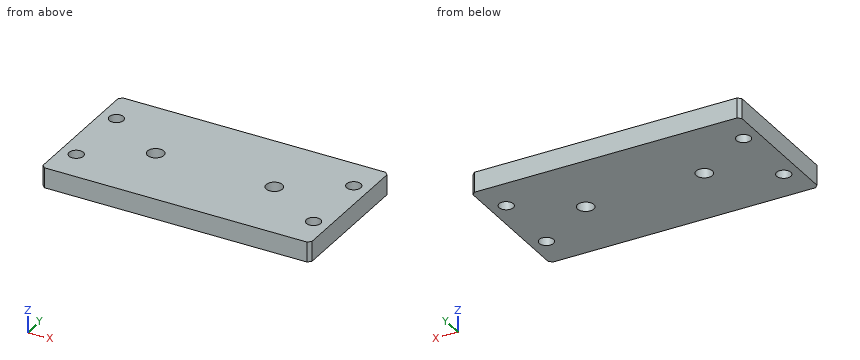
```python
from build123d import *

# Parameters (mm, degrees)
F0_W     = 170
F0_H     = 88
F0_R     = 4.5
F1_DEPTH = 6.35
F2_SIZE  = 2
F4_D     = 10.3


with BuildPart() as f1:
    # F0 (on Top) → F1 (new body, symmetric)
    with BuildSketch(Plane.XY):
        Rectangle(F0_W, F0_H)
        with Locations((-75, -22.5)):
            Circle(F0_R, mode=Mode.SUBTRACT)
        with Locations((75, -22.5)):
            Circle(F0_R, mode=Mode.SUBTRACT)
        with Locations((-75, 22.5)):
            Circle(F0_R, mode=Mode.SUBTRACT)
        with Locations((75, 22.5)):
            Circle(F0_R, mode=Mode.SUBTRACT)
    extrude(amount=F1_DEPTH, both=True)

    # F2
    f2_edges = [f1.edges().sort_by_distance(p)[0] for p in [
        (85, 44, 0),
        (85, -44, 0),
        (-85, 44, 0),
        (-85, -44, 0),
    ]]
    chamfer(f2_edges, length=F2_SIZE)

    # F4 (through all)
    with Locations(Plane.XY.offset(6.35)):
        with Locations((-37.5, 0), (37.5, 0)):
            Hole(F4_D / 2)


solid = f1.part
```
Source: CAD feature listing. Evaluate the final solid. Frame: model axes, mm. Give positions to 0.01 mm unless a question says otherwise; leave off trailing zeros. Order: outer loops, then holes, each group sorted by start corner. A loop starts at its lowest first (then second) coordinate and runs counter-clockwise, first axis right, second up.
(1) Section query A-A (x = 37.5). Return the cut outline in (y, z).
(2) Section query B-B (y = 0). Return the cut outline in (x, z).
(3) Contact query for flat-ended pins moving along their axis: P1, Ø8, axis at x = -75, y = 22.5, coming from the -Z side; P2, Ø10.5, axis at x = 75, y = -22.5, coming from the +Z side. Output: stop coordinate, or through.
(4) Section query C-C (z = -3.25). Return the cut outline in (x, y), plus the area to 3 significant figures.
(5) Material intervals for line 1 along Y through (x, z) = (-75, -1.25); line 2 along Y through (x, z) = (37.5, -1); line 3 along X through (y, z) = (18.5, -3), sorted ascending.
(6) Section query D-D (x = 75). Return the cut outline in (y, z).
Outcome:
1. outline: (-44, -6.35) - (-5.15, -6.35) - (-5.15, 6.35) - (-44, 6.35) - close; (5.15, -6.35) - (44, -6.35) - (44, 6.35) - (5.15, 6.35) - close
2. outline: (-85, -6.35) - (-42.65, -6.35) - (-42.65, 6.35) - (-85, 6.35) - close; (-32.35, -6.35) - (32.35, -6.35) - (32.35, 6.35) - (-32.35, 6.35) - close; (42.65, -6.35) - (85, -6.35) - (85, 6.35) - (42.65, 6.35) - close
3. P1: passes through
3. P2: stops at z = 6.35
4. outline: (-85, -42) - (-83, -44) - (83, -44) - (85, -42) - (85, 42) - (83, 44) - (-83, 44) - (-85, 42) - close; hole circle Ø9 at (-75, -22.5); hole circle Ø9 at (-75, 22.5); hole circle Ø10.3 at (-37.5, 0); hole circle Ø10.3 at (37.5, 0); hole circle Ø9 at (75, -22.5); hole circle Ø9 at (75, 22.5)
4. area: 14,500 mm2
5. line 1: y = -44 to -27, -18 to 18, 27 to 44
5. line 2: y = -44 to -5.15, 5.15 to 44
5. line 3: x = -85 to -77.06, -72.94 to 72.94, 77.06 to 85
6. outline: (-44, -6.35) - (-27, -6.35) - (-27, 6.35) - (-44, 6.35) - close; (-18, -6.35) - (18, -6.35) - (18, 6.35) - (-18, 6.35) - close; (27, -6.35) - (44, -6.35) - (44, 6.35) - (27, 6.35) - close
